from build123d import *

# Parameters (mm, degrees)
F1_DEPTH  = 8
F3_ANGLE  = 33
F6_DEPTH  = 26.5
F7_W      = 18.4942251071
F7_H      = 9.6429027617
F8_DEPTH  = 25
F9_SIZE   = 0.5
F10_SIZE2 = 2.99999
F10_SIZE  = 7.99999
F11_SIZE  = 0.46
F12_SIZE  = 0.475
F13_SIZE  = 0.56


# Not quite as in the source:
# - a fillet or chamfer is up to 0.001 mm smaller than in the source, because OpenCascade refuses the exact size


with BuildPart() as f1:
    # F0 (on Front) → F1 (new body)
    with BuildSketch(Plane.XZ):
        Polygon((-2.45, 5.9), (-4.9, 0), (4.9, 0), (2.45, 5.9), align=None)
    extrude(amount=F1_DEPTH)

    # F2 (on face) → F3 (revolve)
    with BuildSketch(Plane.XZ.offset(8)):
        Polygon((4.9, 0), (2.45, 5.9), (-2.45, 5.9), (-4.9, 0), align=None)
    revolve(axis=Axis((0, -8, 5.9), (-1, 0, 0)), revolution_arc=F3_ANGLE)

    # F4 (on face) → F6 (join)
    with BuildSketch(Plane(origin=(0, -8.3219056723, 5.4043087335), x_dir=(1, 0, 0), z_dir=(0, -0.8386705679, 0.544639035))):
        Polygon((-4.9, -5.3089559292), (4.9, -5.3089559292), (2.45, 0.5910440708), (-2.45, 0.5910440708), align=None)
    extrude(amount=F6_DEPTH)

    # F7 (on Top) → F8 (cut)
    with BuildSketch(Plane.XY):
        with Locations((0.8348836564, -34.8214513808)):
            Rectangle(F7_W, F7_H)
    extrude(amount=F8_DEPTH, mode=Mode.SUBTRACT)

    # F9
    f9_edges = [f1.edges().sort_by_distance(p)[0] for p in [
        (4.9, -4, 0),
        (-4.9, -4, 0),
    ]]
    chamfer(f9_edges, length=F9_SIZE)

    # F10 (size 8 and 3 in the source; OpenCascade refuses exactly that, so slightly less here)
    f10_edges = [f1.edges().sort_by_distance(p)[0] for p in [
        (0, 0, 5.9),
    ]]
    f10_side = f1.faces().sort_by_distance((0, -4, 5.9))[0]
    chamfer(f10_edges, length=F10_SIZE, length2=F10_SIZE2, reference=f10_side)

    # F11
    f11_edges = [f1.edges().sort_by_distance(p)[0] for p in [
        (0, 0, 0),
    ]]
    chamfer(f11_edges, length=F11_SIZE)

    # F12
    f12_edges = [f1.edges().sort_by_distance(p)[0] for p in [
        (-3.579124, -30, 16.944794),
        (3.579124, -30, 16.944794),
    ]]
    chamfer(f12_edges, length=F12_SIZE)

    # F13
    f13_edges = [f1.edges().sort_by_distance(p)[0] for p in [
        (0, -30, 20.186967),
    ]]
    chamfer(f13_edges, length=F13_SIZE)


solid = f1.part
Part model, mm, in its own coordinate system. A direction names the side the tool comes from. Coordinates: 2 decimals unless noted, no trailing zeros. Order: outer loops, then holes, each group sorted by start corner. A loop starts at its lowest first (then second) coordinate and runs counter-clockwise, first axis right, second up. Notation, with made-up numbers: M 78.5,4.25 L 134.5,4.25 A26 cw 134.5,35.25 Z; hole C 89,-11 d4. An arc over 180 degrees is marked long. Use a Markdown table: item, result.
(1) Tool access for faces 1 (the flat face through (-3.814, -4.833, 2.615)), 2 (the flat face through (0.052, -3.944, 4.379)), 3 (the flat face through (3.846, -4.833, 2.539)): list every direction of +Z, -Z, +X, -X, +Y, -Y with a clear straight run to the whole face (end or side of a thin tool).
A:
| item | result |
|---|---|
| face 1 | +Z, -X, +Y |
| face 2 | +Z, +X, -X, +Y |
| face 3 | +Z, +X, +Y |
(2) Cut at D-D on x = -4. Write the cut outline in (y, z), then the cut area to 3 significant figures.
A:
| item | result |
|---|---|
| outline | M -30,13.15 L -11.21,0.95 A5.9 ccw -8,0 L -0.46,0 L 0,0.46 L 0,2.17 L -8,2.17 A3.73 cw -10.03,2.77 L -29.54,15.43 L -30,14.29 Z |
| area | 73.0 mm^2 |
(3) Cut at C-C on y = -2.75. Write the cut outline in (x, z).
A:
| item | result |
|---|---|
| outline | M -4.71,0.46 L -4.4,0 L 4.4,0 L 4.71,0.46 L 3.27,3.93 L -3.27,3.93 Z |
(4) Cut at B-B on z = 8.25. Write the cut outline in (x, y).
A:
| item | result |
|---|---|
| outline | M -4.71,-21.6 L -4.4,-22.45 L 4.4,-22.45 L 4.71,-21.6 L 2.45,-11.62 L -2.45,-11.62 Z |
(5) Flat gauge pins, fed straight in: pin 1 (5 mm diameter, centred on x = -2.5, y = -18, fed in from -Z); pin 2 (2 mm diameter, centred on x = 2.5, z = 3, fed in from -Y); pin 3 (5 mm diameter, centred on x = 1, y = -24, fed in from +Z). Where does each tip first touch, or does it go through?
A:
| item | result |
|---|---|
| pin 1 | stops at z = 3.74 |
| pin 2 | stops at y = -15.91 |
| pin 3 | stops at z = 17.91 |
(6) Probe L1, parallel to Z at x = 1.25, y = -12; L2, parallel to Z at x = 2.25, y = -9.25; L3, parallel to X at y = -11.25, z = 6.25. List the from-to ranges inside material, lowest first.
A:
| item | result |
|---|---|
| L1 | z = 1.46 to 8.5 |
| L2 | z = 0.13 to 6.71 |
| L3 | x = -3.06 to 3.06 |
